Work out the finished part from the listing and answer in its coordinate system (mm). A direction names the side the tool comes from. Coordinates: 2 decimals unless noted, no trailing zeros. Write each loop counter-clockwise with the first axis right and the second up, starting at its lowest first coordinate (ties: lowest second). Pieces come first, ordered by that corner, then holes. Notation, with made-up numbers: (2.5, -8) - (39.5, -8) arc R27 ccw to (39.5, 30) - close; hole circle Ø3 at (-20.75, -18). An arc over 180 degrees is marked (long way). One line per item, written item: value.
```python
from build123d import *

# Parameters (mm, degrees)
SKETCH1_W           = 41
SKETCH1_H           = 61
BOSS_EXTRUDE1_DEPTH = 3
SKETCH2_W           = 21
SKETCH2_H           = 41
CUT_EXTRUDE1_DEPTH  = 3
SKETCH3_R           = 2
CUT_EXTRUDE2_DEPTH  = 3
SKETCH4_R           = 2
CUT_EXTRUDE3_DEPTH  = 10


with BuildPart() as part:
    # Sketch1 → Boss-Extrude1 (new body)
    with BuildSketch(Plane.XY):
        with Locations((20.5, -30.5)):
            Rectangle(SKETCH1_W, SKETCH1_H)
    extrude(amount=BOSS_EXTRUDE1_DEPTH)

    # Sketch2 → Cut-Extrude1 (cut)
    with BuildSketch(Plane.XY.offset(3)):
        with Locations((20.5, -30.5)):
            Rectangle(SKETCH2_W, SKETCH2_H)
    extrude(amount=-CUT_EXTRUDE1_DEPTH, mode=Mode.SUBTRACT)

    # Sketch3 → Cut-Extrude2 (cut)
    with BuildSketch(Plane.XY.offset(3)):
        with Locations((36, -25.5)):
            Circle(SKETCH3_R)
        with Locations((5, -25.5)):
            Circle(SKETCH3_R)
    extrude(amount=-CUT_EXTRUDE2_DEPTH, mode=Mode.SUBTRACT)

    # Sketch4 → Cut-Extrude3 (cut)
    with BuildSketch(Plane.XY.offset(3)):
        with Locations((20.5, -5)):
            Circle(SKETCH4_R)
        with Locations((20.5, -56)):
            Circle(SKETCH4_R)
    extrude(amount=-CUT_EXTRUDE3_DEPTH, mode=Mode.SUBTRACT)


solid = part.part
```
Item 1: Section A-A, the plane x = 20.5 is taken. Determine the outline of the cut face in (y, z).
Evaluation:
outline: (-61, 0) - (-58, 0) - (-58, 3) - (-61, 3) - close; (-54, 0) - (-51, 0) - (-51, 3) - (-54, 3) - close; (-10, 0) - (-7, 0) - (-7, 3) - (-10, 3) - close; (-3, 0) - (0, 0) - (0, 3) - (-3, 3) - close
Item 2: Which of the six approach directions +Z, -Z, +X, -X, +Y, -Y give full straight-line access (tool end or side, diameter ignored) to faces 5 (the face through (20, -51, 2)), 6 (the face through (41, -31, 1))?
Evaluation:
face 5: +Z, -Z
face 6: +Z, -Z, +X, +Y, -Y
Item 3: Given pin 1 (2 mm diameter, centred on x = 32.5, y = -54.5, fed in from -Z), flat-ended and moving along its own axis, determine where the tip first touches the part or whether it passes through.
Evaluation:
pin 1: stops at z = 0
Item 4: Section C-C, the plane y = -25.5 is taken. Determine the outline of the cut face in (x, z), then the cut area to 3 significant figures.
Evaluation:
outline: (0, 0) - (3, 0) - (3, 3) - (0, 3) - close; (7, 0) - (10, 0) - (10, 3) - (7, 3) - close; (31, 0) - (34, 0) - (34, 3) - (31, 3) - close; (38, 0) - (41, 0) - (41, 3) - (38, 3) - close
area: 36.0 mm2
Item 5: Determine the mould class of faces 1 (the face through (10, -31, 2)), 2 (the face through (20, 0, 1)), 3 (the face through (18.9, -6.2, 1.5)), 4 (the face through (0, -31, 1)) for opening direction X: +X half, -X half, draft (parallel to the pull), parting line (faces both ways), or undercut.
Evaluation:
face 1: undercut
face 2: draft
face 3: undercut
face 4: -X half
Item 6: Section B-B, the plane y = -14 is taken. Determine the outline of the cut face in (x, z).
Evaluation:
outline: (0, 0) - (10, 0) - (10, 3) - (0, 3) - close; (31, 0) - (41, 0) - (41, 3) - (31, 3) - close
Item 7: Section D-D, the plane x = 36 is taken. Determine the outline of the cut face in (y, z).
Evaluation:
outline: (-61, 0) - (-27.5, 0) - (-27.5, 3) - (-61, 3) - close; (-23.5, 0) - (0, 0) - (0, 3) - (-23.5, 3) - close
Item 8: Consider probe 1 along Y at (x, z) = (20.5, 0.6); probe 2 along Y at (x, z) = (26, 2.8); probe 3 along Y at (x, z) = (36, 0.75). Determine where each line is inside the solid, lowest interval first.
Evaluation:
probe 1: y = -61 to -58, -54 to -51, -10 to -7, -3 to 0
probe 2: y = -61 to -51, -10 to 0
probe 3: y = -61 to -27.5, -23.5 to 0
